Autodesk Fusion 360 part; units mm, degrees
sketch "Sketch1" plane through (0, 0, 0) normal (0, 0, 1) x (1, 0, 0)
  line L0 (68.38, -47.235) -> (-68.38, -47.235)
  line L1 (-68.38, -47.235) -> (-68.38, 47.235)
  line L2 (-68.38, 47.235) -> (68.38, 47.235)
  line L3 (68.38, 47.235) -> (68.38, -47.235)
  line L4 (68.38, -47.235) -> (-68.38, 47.235) construction
  line L5 (-68.38, -47.235) -> (68.38, 47.235) construction
  line L6 (-48.38, 47.235) -> (-58.38, 47.235)
  line L7 (-58.38, 47.235) -> (-58.38, 57.235)
  line L8 (-58.38, 57.235) -> (-48.38, 57.235)
  line L9 (-48.38, 57.235) -> (-48.38, 47.235)
  line L10 (-48.38, 47.235) -> (-58.38, 57.235) construction
  line L11 (-58.38, 47.235) -> (-48.38, 57.235) construction
  line L12 (48.38, 57.235) -> (58.38, 57.235)
  line L13 (48.38, 47.235) -> (48.38, 57.235)
  line L14 (58.38, 57.235) -> (58.38, 47.235)
  line L15 (58.38, 47.235) -> (48.38, 47.235)
  line L16 (48.38, -57.235) -> (48.38, -47.235)
  line L17 (48.38, -47.235) -> (58.38, -47.235)
  line L18 (58.38, -47.235) -> (58.38, -57.235)
  line L19 (48.38, -57.235) -> (58.38, -57.235)
  line L20 (-58.38, -57.235) -> (-58.38, -47.235)
  line L21 (-58.38, -47.235) -> (-48.38, -47.235)
  line L22 (-48.38, -47.235) -> (-48.38, -57.235)
  line L23 (-48.38, -57.235) -> (-58.38, -57.235)
  point P0 (-53.38, 52.235)
  dimension "d1" = 136.76
  dimension "d2" = 94.47
  dimension "d3" = 10
  dimension "d4" = 10
  dimension "d6" = 10
  dimension "d7" = 10
extrude "Extrude1" add sketch "Sketch1" along normal blind 10 and the other way blind 0
ref_plane "WorkPlane1" through (0, 0, 10) normal (0, 0, 1) x (1, 0, 0)
sketch "Sketch2" plane through (0, 0, 10) normal (0, 0, 1) x (1, 0, 0)
  line L0 (62.5, -41.5) -> (-62.5, -41.5)
  line L1 (-62.5, -41.5) -> (-62.5, 41.5)
  line L2 (-62.5, 41.5) -> (62.5, 41.5)
  line L3 (62.5, 41.5) -> (62.5, -41.5)
  line L4 (62.5, -41.5) -> (-62.5, 41.5) construction
  line L5 (-62.5, -41.5) -> (62.5, 41.5) construction
  line L6 (-62.5, -41.5) -> (-62.5, 34.9)
  line L7 (62.5, 41.5) -> (-55.8, 41.5)
  line L8 (-62.5, 34.9) -> (-55.8, 41.5)
  dimension "d13" = 125
  dimension "d14" = 83
  dimension "d15" = 76.4
  dimension "d16" = 118.3
extrude "Extrude2" cut sketch "Sketch2" against normal blind 8 contours L0 L1 L2 L3 L6 L7 L8
ref_plane "WorkPlane2" through (0, 0, 10) normal (0, 0, 1) x (1, 0, 0)
sketch "Sketch3" plane through (0, 0, 10) normal (0, 0, 1) x (1, 0, 0)
  circle A0 centre (-53.3802, 52.2353) radius 3.25
  circle A1 centre (53.38, 52.2349) radius 3.25
  circle A2 centre (53.3799, -52.2347) radius 3.25
  circle A3 centre (-53.3802, -52.2349) radius 3.25
  dimension "d20" = 6.5
  dimension "d21" = 6.5
  dimension "d22" = 6.5
  dimension "d23" = 6.5
extrude "Extrude3" cut sketch "Sketch3" against normal blind 10
fillet "Fillet1" radius 5 4 edges at (68.38, -47.235, 5) (68.38, 47.235, 5) (-68.38, -47.235, 5) (-68.38, 47.235, 5)
fillet "Fillet2" radius 2 16 edges at (58.38, -47.235, 5) (58.38, -57.235, 5) (48.38, -57.235, 5) (58.38, 57.235, 5) (-48.38, -47.235, 5) (-48.38, -57.235, 5) (-58.38, -57.235, 5) (-48.38, 57.235, 5) (58.38, 47.235, 5) (-48.38, 47.235, 5) (-58.38, 57.235, 5) (48.38, 57.235, 5) (48.38, 47.235, 5) (-58.38, 47.235, 5) (48.38, -47.235, 5) (-58.38, -47.235, 5)
extrude "Extrude4" add 1 faces at (-18.6, -13.8333, 2) along direction (0, 0, 1) blind 8
ref_plane "WorkPlane3" through (0, 0, 10) normal (0, 0, 1) x (1, 0, 0)
sketch "Sketch4" plane through (0, 0, 10) normal (0, 0, 1) x (1, 0, 0)
  line L0 (63, -42) -> (-63, -42)
  line L1 (-63, -42) -> (-63, 42)
  line L2 (-63, 42) -> (63, 42)
  line L3 (63, 42) -> (63, -42)
  line L4 (63, -42) -> (-63, 42) construction
  line L5 (-63, -42) -> (63, 42) construction
  line L6 (63, -42) -> (63, 34.4)
  line L7 (-63, 42) -> (55.3, 42)
  line L8 (55.3, 42) -> (63, 34.4)
  dimension "d31" = 126
  dimension "d32" = 84
  dimension "d33" = 76.4
  dimension "d34" = 118.3
extrude "Extrude6" cut sketch "Sketch4" against normal blind 8 contours L0 L1 L2 L3 L6 L7 L8
extrude "Extrude5" cut sketch "Sketch4" against normal blind 8 contours L0 L1 L2 L3 L6 L7 L8
For this review, take the finished solid that the model builds, in its own axes (mm). A direction names the side the tool comes from. Give positions to 0.01 mm unless a question says otherwise; leave off trailing zeros. Loops run counter-clockwise (first coordinate to the right, second up) from the corner with the lowest first, then second, coordinate; pieces in that order, holes last. Notation, with made-up numbers: M -6,9 L 36,9 A12 cw 36,24 Z; hole C 36.5,0 d3. An arc over 180 degrees is marked long. Put each result on its own line as item: value. Start each with the question number.
(1) The part is to be moulded in two halves that separate along Y. For faces 1 (the flat face through (59.1, 38.25, 6.06)), 2 (the flat face through (-68.38, -1, 5)), 3 (the flat face through (62, -47.235, 5)), 4 (the cylindrical face through (-51.633, 54.976, 5.07)), say which applies: +Y half, -Y half, draft (parallel to the pull), parting line (faces both ways), or undercut.
(2) Add section C-C, the plane y = 2. Write out the cut boundary in (x, z), then the cut area to 3 significant figures.
(3) Add section B-B, the plane x = -3. Write out the cut boundary in (y, z) (3 decimals), then the cut area to 3 significant figures.
(4) Machinability: for faces 5 (the flat face through (-48.38, -52, 5)), 6 (the flat face through (-62, -47.235, 5)), 7 (the flat face through (-1, 47.235, 5)), which of the approach directions +Z, -Z, +X, -X, +Y, -Y give a long, thin tool a straight path to every point of the face, cutting with its end or side? Answer none if there is none.
(5) Wall thickness on L1, parallel to Y at x = 53.38, z = 3.5 (3 decimals); L2, parallel to X at y = -52, z = 1.75; L3, parallel to Y at x = 0, z = 6.75 (3 decimals): over which ranges is each line inside the solid? List them lowest first.
(6) Add section A-A, the plane x = 53.38. Write out the cut boundary in (y, z) (3 decimals).
(7) Add section D-D, the plane z = 4. Give the number of separate pieces and of enclosed holes in the cut face, then the cut area to 3 significant figures.
(8) For pin 1 (1.8 mm diameter, centred on y = 53, z = 5.5, fed in from -X); pin 2 (6 mm diameter, centred on x = -39.5, z = 6.5, fed in from -Y) (3 decimals); pin 3 (2.5 mm diameter, centred on x = 18.5, z = 4.5, fed in from +Y) (3 decimals), all flat-tipped, find the tip position at first contact; note any pin that passes through.
Result:
1. face 1: undercut
1. face 2: draft
1. face 3: -Y half
1. face 4: undercut
2. outline: M -68.38,0 L 68.38,0 L 68.38,10 L 63,10 L 63,2 L -63,2 L -63,10 L -68.38,10 Z
2. area: 360 mm^2
3. outline: M -47.235,0 L 47.235,0 L 47.235,10 L 42,10 L 42,2 L -42,2 L -42,10 L -47.235,10 Z
3. area: 273 mm^2
4. face 5: +Z, -Z, -Y
4. face 6: +Z, -Z, -X, -Y
4. face 7: +Z, -Z, +Y
5. L1: y = -57.235 to -55.485, -48.985 to -42, 42 to 48.985, 55.485 to 57.235
5. L2: x = -58.38 to -56.62, -50.14 to -48.38, 48.38 to 50.14, 56.62 to 58.38
5. L3: y = -47.235 to -42, 42 to 47.235
6. outline: M -57.235,0 L -55.485,0 L -55.485,10 L -57.235,10 Z; M -48.985,0 L 48.985,0 L 48.985,10 L 42,10 L 42,2 L -42,2 L -42,10 L -48.985,10 Z; M 55.485,0 L 57.235,0 L 57.235,10 L 55.485,10 Z
7. separate pieces: 1
7. enclosed holes: 5
7. area: 2,610 mm^2
8. pin 1: stops at x = -58.38
8. pin 2: stops at y = -47.235
8. pin 3: stops at y = 47.235
